Geometry: see drawing. Coordinates: mm, zero at the bounding-box minimum. Round coordinates to 2 decimals unless told otherwise and drop trailing zeros. Order: outer loops, then holes, each group sorted by start corner. A loop starts at its lowest first (then second) coordinate and runs counter-clockwise, first axis right, second up. Notation, with made-up numbers: M 52,33.25 L 79,33.25 A12 ccw 79,56.25 Z; hole C 34.25,26.5 d9. An arc over 180 degrees is marked long. Answer in a Markdown table with one row per item. Add a question column.
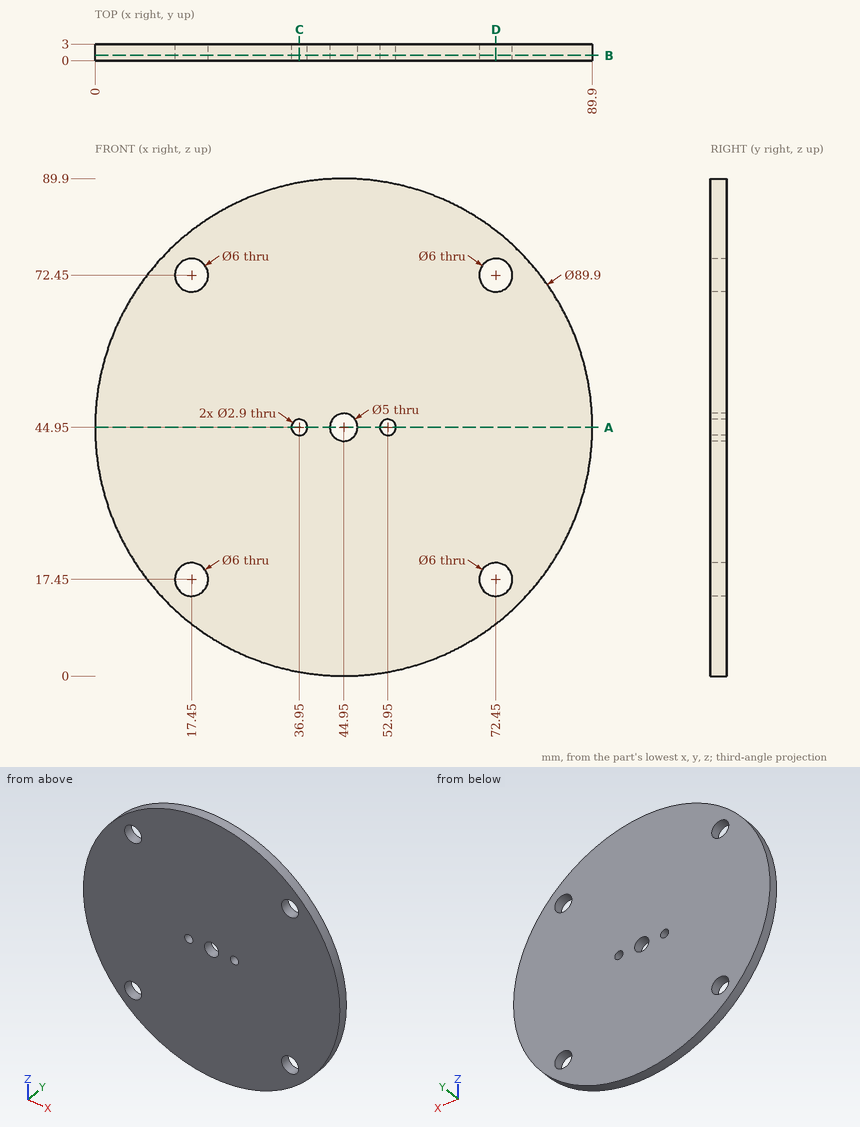
(1) Cut plane C-C (x = 36.95). Return loops of the section in (y, z).
(2) Pin query (flat end, axial travel): pin 1 (3 mm diameter, centred on x = 44.95, z = 44.95, fed in from -Y); pin 2 (1.5 mm diameter, centred on y = 1, z = 41, fed in from -X). Return the tip coordinate at first contact, or that it passes through.
(3) Line query: line 1 (Z direction, x = 44.95, y = 1); line 2 (Z direction, x = 71.5, y = 1.45); line 3 (X direction, y = 0.7, z = 17). Output: solid intervals per line, ascending. Write a range as from..to.
(4) Cut plane D-D (x = 72.45). Return loops of the section in (y, z).
(5) Cut plane A-A (z = 44.95). Return loops of the section in (x, y), and give its area (3 significant figures).
(6) Cut plane B-B (y = 0.95). Return loops of the section in (x, z).
Answer list:
| question | item | result |
|---|---|---|
| 1 | outline | M 0,0.72 L 3,0.72 L 3,43.5 L 0,43.5 Z; M 0,46.4 L 3,46.4 L 3,89.18 L 0,89.18 Z |
| 2 | pin 1 | through |
| 2 | pin 2 | x = 0.11 |
| 3 | line 1 | 0..42.45, 47.45..89.9 |
| 3 | line 2 | 8.68..14.6, 20.3..69.6, 75.3..81.22 |
| 3 | line 3 | 9.75..14.48, 20.42..69.48, 75.42..80.15 |
| 4 | outline | M 0,9.39 L 3,9.39 L 3,14.45 L 0,14.45 Z; M 0,20.45 L 3,20.45 L 3,69.45 L 0,69.45 Z; M 0,75.45 L 3,75.45 L 3,80.51 L 0,80.51 Z |
| 5 | outline | M 0,0 L 35.5,0 L 35.5,3 L 0,3 Z; M 38.4,0 L 42.45,0 L 42.45,3 L 38.4,3 Z; M 47.45,0 L 51.5,0 L 51.5,3 L 47.45,3 Z; M 54.4,0 L 89.9,0 L 89.9,3 L 54.4,3 Z |
| 5 | area | 237 mm² |
| 6 | outline | C 44.95,44.95 d89.9; hole C 17.45,17.45 d6; hole C 17.45,72.45 d6; hole C 36.95,44.95 d2.9; hole C 44.95,44.95 d5; hole C 52.95,44.95 d2.9; hole C 72.45,17.45 d6; hole C 72.45,72.45 d6 |
